Autodesk Inventor part; units mm, degrees
ref_plane "Arbeitsebene1" through (0, 40, 0) normal (0, -1, 0) x (1, 0, 0)
ref_plane "YZ Plane" through (0, 0, 0) normal (1, 0, 0) x (0, 1, 0)
ref_plane "XZ Plane" through (0, 0, 0) normal (0, 1, 0) x (-1, 0, 0)
sketch "Skizze1" plane through (0, 0, 0) normal (0, 1, 0) x (-1, 0, 0)
  circle A0 centre (0, 0) radius 15
  dimension "d0" = 30
sketch "Skizze2" plane through (0, 0, 0) normal (1, 0, 0) x (0, 1, 0)
  line L0 (0, 0) -> (122.9469, 0)
  line L1 (136.6277, 2.4123) -> (252.16, 44.4626)
  arc A0 (122.9469, 0) -> (136.6277, 2.4123) centre (122.9469, 40) ccw
  point P0 (130, 0)
  dimension "d1" = 160
  dimension "d2" = 130
  dimension "d3" = 130
  dimension "d4" = 40
sweep "Sweeping1" add profiles "Skizze1" path "Skizze2"
sketch "Skizze3" plane through (0, 0, 0) normal (1, 0, 0) x (0, 1, 0)
  line L0 (257.2903, 30.3672) -> (247.0297, 58.558)
  line L1 (141.758, -11.6831) -> (131.4974, 16.5077)
  line L2 (257.2903, 30.3672) -> (247.0297, 58.558)
  circle A0 centre (252.16, 44.4626) radius 15
  point P0 (0, 0)
extrude "Extrusion1" add sketch "Skizze3" along normal mid plane 200
ref_plane "Arbeitsebene1" through (0, 40, 0) normal (0, -1, 0) x (1, 0, 0)
sketch "Skizze4" plane through (0, 40, 0) normal (0, -1, 0) x (1, 0, 0)
  circle A0 centre (0, 0) radius 25
  dimension "d10" = 50
extrude "Extrusion2" add sketch "Skizze4" along normal blind 3
sketch "Skizze5" plane through (100, 252.16, 44.4626) normal (1, 0, 0) x (0, 0, -1)
  circle A0 centre (0, 0) radius 14
  point P0 (44.4626, -252.16)
  dimension "d13" = 28
extrude "Extrusion3" add sketch "Skizze5" along normal blind 2
sketch "Skizze6" plane through (-100, 252.16, 44.4626) normal (-1, 0, 0) x (0, 0, 1)
  circle A0 centre (0, 0) radius 14
  point P0 (-44.4626, -252.16)
  dimension "d16" = 28
extrude "Extrusion4" add sketch "Skizze6" along normal blind 2
chamfer "Fase1" distance 1 angle 45 2 edges at (102, 252.16, 58.4626) (-102, 252.16, 30.4626)
properties part number "Bootsklampe Metall"
Model file for the job. Use its own axes, mm. A direction names the side the tool comes from. Give positions to 0.01 mm unless a question says otherwise; leave off trailing zeros. Loops run counter-clockwise (first coordinate to the right, second up) from the corner with the lowest first, then second, coordinate; pieces in that order, holes last. Notation, with made-up numbers: (-18, -26) - (40, -26) arc R29 ccw to (40, -1) - close; hole circle Ø10 at (46, 35.5). An arc over 180 degrees is marked (long way). One line per item, written item: value. Start each with the question number.
1. Pin check, flat tips, straight feed: pin 1 (12 mm diameter, centred on x = 18.5, y = 137.5, fed in from +Z); pin 2 (4 mm diameter, centred on x = -40.5, z = 32.5, fed in from +Y); pin 3 (3 mm diameter, centred on x = 0, z = 20.5, fed in from -Y). Stop position of each tip, or through.
2. Probe L1, parallel to X at y = 35.5, z = 1; L2, parallel to Y at x = -68, z = 43; L3, parallel to Y at x = -18.5, z = 38. List the from-to ranges inside material, lowest first. Write a range as from..to.
3. Which spindle directions (+Z, -Z, +X, -X, +Y, -Y) get a long thin tool onto all of the face, cutting with end or side? Do faces 5 (the flat face through (-100, 245, 57)), 6 (the flat face through (11, 37, -11)), 7 (the flat face through (100, 245, 57)), 8 (the cylindrical face through (1.4, 266.467, 48.968)). Say none if no direction does.
4. Pull direction Y, two halves, no side cores. Call faces 1 (the flat face through (0, 0, 0)), 2 (the cylindrical face through (14.985, 82.054, 0.66)), 3 (the flat face through (11, 40, -11)), 4 (the flat face through (102, 252, 45)): pulls with the +Y half, pulls with the -Y half, needs draft (parallel to the pull), parting line crosses it, or undercut.
5. Slice it at A-A (y = 94). List the corners of the cut face in (x, z), plus the area to 3 significant figures.
Solution:
1. pin 1: stops at z = 11.79
1. pin 2: stops at y = 263.37
1. pin 3: stops at y = 37
2. L1: x = -14.97..14.97
2. L2: y = 237.23..267.09
2. L3: y = 238.62..265.7
3. face 5: -X
3. face 6: -Y
3. face 7: +X
3. face 8: none
4. face 1: pulls with the -Y half
4. face 2: undercut
4. face 3: undercut
4. face 4: needs draft
5. outline: circle Ø30 at (0, 0)
5. area: 707 mm^2
